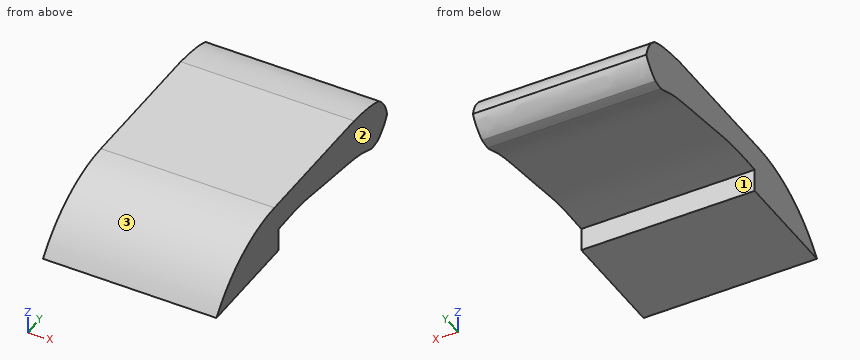
```python
from build123d import *

# Parameters (mm, degrees)
F0_W        = 67
F0_H        = 20
F1_DEPTH    = 118
F3_T1_DEPTH = 267
F4_R        = 15
F5_T1_DEPTH = 122.9016994375
F6_DEPTH    = 67.001
F7_R        = 0.0241421356


# Not quite as in the source:
# - a fillet or chamfer that OpenCascade refuses, or shapes differently, is made with other operations: its cross-section is extruded or revolved along the edge and cut away or added


with BuildPart() as f1:
    # F0 (on Front) → F1 (new body)
    with BuildSketch(Plane.XZ):
        with Locations((6.337375957, -47.2683286667)):
            Rectangle(F0_W, F0_H)
    extrude(amount=F1_DEPTH)

    # F3: fillet of radius 50 on 1 edges, made by hand

    # F3_s2 → F3_t1 (cut)
    with BuildSketch(Plane.YZ.offset(-127.162624043)):
        with BuildLine():
            ThreePointArc((-78, -37.2683286667), (-100.360679775, -42.5469691167), (-118, -57.2683286667))
            Line((-118, -57.2683286667), (-118, -37.2683286667))
            Line((-118, -37.2683286667), (-78, -37.2683286667))
        make_face()
    extrude(amount=F3_T1_DEPTH, mode=Mode.SUBTRACT)

    # F4
    f4_edges = [f1.edges().sort_by_distance(p)[0] for p in [
        (6.337376, -78, -37.268329),
        (6.337376, 0, -37.268329),
    ]]
    fillet(f4_edges, radius=F4_R)

    # F5: fillet of radius 15 on 1 edges, made by hand

    # F5_s2 → F5_t1 (cut)
    with BuildSketch(Plane.YZ.offset(-55.1134737617)):
        with BuildLine():
            ThreePointArc((0, -52.2683286667), (-5.0566155305, -55.9613926043), (-11.1803398875, -57.2683286667))
            Line((-11.1803398875, -57.2683286667), (0, -57.2683286667))
            Line((0, -57.2683286667), (0, -52.2683286667))
        make_face()
    extrude(amount=F5_T1_DEPTH, mode=Mode.SUBTRACT)

    # F2 (on face) → F6 (cut, through all)
    with BuildSketch(Plane.YZ.offset(39.837375957)):
        with BuildLine():
            Line((-75, -48.2683286667), (-75, -57.2683286667))
            Line((-75, -57.2683286667), (-10.1939006259, -57.2683286667))
            add(Edge.make_bspline(
                [(-75, -48.2683286667), (-69.6300083872, -48.0932397516), (-59.1455400015, -47.7513929988), (-45.397034891, -50.3214203198), (-27.6071602735, -52.6118617406), (-16.9114345494, -54.5205994978), (-11.9954400696, -57.0260607697), (-10.1939006259, -57.2683286667)],
                knots=[0, 0, 0, 0, 0.1168750086, 0.2281888728, 0.353191241, 0.4546285253, 0.5170585623, 0.5170585623, 0.5170585623, 0.5170585623], degree=3))
        make_face()
        with BuildLine():
            add(Edge.make_bspline(
                [(-8.5831200704, -57.2683286667), (-6.3182593416, -56.9222504863), (-2.2304747887, -53.2529046852), (-0.154748351, -50.0842721126), (0, -48.2683286667)],
                knots=[0.5358591005, 0.5358591005, 0.5358591005, 0.5358591005, 0.6158678035, 0.6848581677, 0.6848581677, 0.6848581677, 0.6848581677], degree=3))
            Line((-8.5831200704, -57.2683286667), (0, -57.2683286667))
            Line((0, -57.2683286667), (0, -48.2683286667))
        make_face()
        with BuildLine():
            Line((0, -37.2683286667), (-22.9681972414, -37.2683286667))
            add(Edge.make_bspline(
                [(0, -47.2220127929), (-0.1541112697, -45.3649297857), (-3.0721745265, -39.2455424759), (-16.4826181453, -37.6339263761), (-22.9681972414, -37.2683286667)],
                knots=[0.69771165, 0.69771165, 0.69771165, 0.69771165, 0.7644699458, 0.8970561658, 0.8970561658, 0.8970561658, 0.8970561658], degree=3))
            Line((0, -47.2220127929), (0, -37.2683286667))
        make_face()
    extrude(amount=-F6_DEPTH, mode=Mode.SUBTRACT)

    # F7
    f7_edges = [f1.edges().sort_by_distance(p)[0] for p in [
        (6.337376, -0.250596, -49.53793),
        (-27.162624, -2.21712, -44.41989),
        (6.337376, -5.891526, -40.350456),
        (39.837376, -2.21712, -44.41989),
    ]]
    fillet(f7_edges, radius=F7_R)


solid = f1.part
```
Geometry check sheet. Reference: the model listing, model coordinates, mm. Face numbers are marked on the shaded views. Round coordinates to 2 decimals unless told otherwise and drop trailing zeros. Order: outer loops, then holes, each group sorted by start corner. A loop starts at its lowest first (then second) coordinate and runs counter-clockwise, first axis right, second up. Notation, with made-up numbers: M 81.5,64 L 98.5,64 A24 ccw 98.5,74 Z; hole C 78,82.25 d11. An arc over 180 degrees is marked long. Write item = value, one per line.
Q1. Depth check by flat-ended pin: pin 1 Ø8 at (x, y) = (9.5, -84.5) entering from +Z; pin 2 Ø1 at (x, z) = (15.5, -51.5) entering from +Y; pin 3 Ø8 at (x, y) = (-11, -45.5) entering from -Z. Enter the tip coordinate at first touch or a pass-through.
Answer block:
pin_1 = -37.33
pin_2 = -0.91
pin_3 = -50.75
Q2. Section check A-A (y = -86). Enter the section's corners in (x, z).
Answer block:
outline = M -27.16,-57.27 L 39.84,-57.27 L 39.84,-37.91 L -27.16,-37.91 Z
Q3. Scan lines: line 1 (Z direction, x = 25, y = -63.5); line 2 (Z direction, x = -18, y = -51.5). Record each from-to range of solid material in increasing order.
Answer block:
line_1 = -48.09 to -37.27
line_2 = -49.2 to -37.27
Q4. Release check for a two-part mould opening along Y. For the marked faces 1, 2 and 3 record: released by +Y, released by -Y, zero draft, split by the parting line, or undercut.
Answer block:
face_1 = undercut
face_2 = zero draft
face_3 = released by -Y
